The listing builds one solid part. Answer for the finished solid, in the listing's coordinates (mm). Face numbers are marked on the shaded views. A direction names the side the tool comes from. Round coordinates to 2 decimals unless told otherwise and drop trailing zeros. Loops run counter-clockwise (first coordinate to the right, second up) from the corner with the lowest first, then second, coordinate; pieces in that order, holes last. Notation, with made-up numbers: (80, 17.25) -> (125, 17.25) arc R4 cw to (125, 23.25) -> close; hole circle Ø9 at (72, 49). An arc over 180 degrees is marked (long way). Use a Markdown table: item, result. Add a question column.
Q1. For a pull along X with two mould halves and no side action, classify the marked faces 1, 2 and 3 as released by +X, released by -X, zero draft, split by the parting line, or undercut.
Q2. Which of the six approach directions +Z, -Z, +X, -X, +Y, -Y give full straight-line access (tool end or side, diameter ignored) to the marked faces 4 and 5?
Q3. Given pin 1 Ø1 at (y, z) = (185, 4.5) entering from +X; pin 2 Ø3 at (y, z) = (179.5, 3.5) entering from +X, each flat-ended and moving along its own axis, determine where each tip first touches the part or whether it passes through.
Q4. Consider line 1 (Y direction, x = 1209, z = 6); line 2 (X direction, y = 195, z = 4.5); line 3 (X direction, y = 187, z = 7). Determine where each line is inside the solid, lowest interval first.
Q5. Section A-A on x = 1208 is taken. Give the vertices of the cut face in (y, z), then the cut area to 3 significant figures.
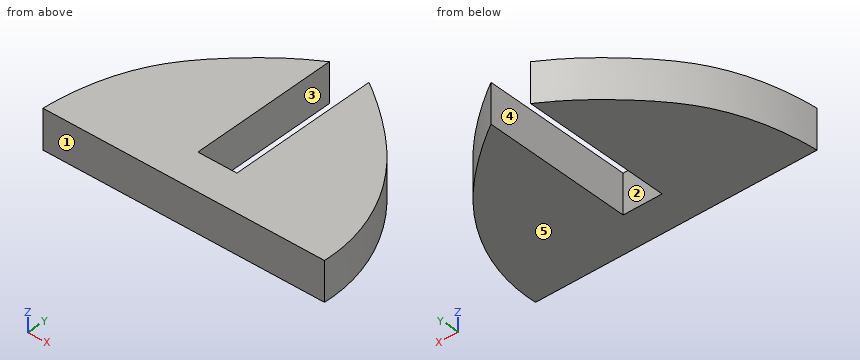
from build123d import *

# Parameters (mm, degrees)
EXTRUDE_1_DEPTH = 8


with BuildPart() as part:
    # 草图1 → 凸台-拉伸1 (new body)
    with BuildSketch(Plane.XY):
        with BuildLine():
            Line((1205.000343889, 200.380448257), (1205.000343889, 170.380448257))
            Line((1205.000343889, 170.380448257), (1212.88866118, 170.380448257))
            Line((1212.88866118, 170.380448257), (1212.88866118, 200.514821588))
            add(Edge.make_bspline(
                [(1212.88866118, 200.514821588), (1213.591796404, 200.102674546), (1216.322248426, 198.206599205), (1221.914919676, 193.964391888), (1232.595967144, 183.625439508), (1237.637966356, 171.491478384), (1237.211883134, 162.95060423)],
                knots=[0.038390069, 0.038390069, 0.038390069, 0.038390069, 0.088763706, 0.237953219, 0.477618195, 1, 1, 1, 1], degree=3))
            Line((1237.211883134, 162.95060423), (1180.232585387, 162.95060423))
            add(Edge.make_bspline(
                [(1205.000343889, 200.380448257), (1203.802132525, 199.644141671), (1199.659392578, 197.029571139), (1193.276793905, 191.438907576), (1183.524062882, 180.866285612), (1180.694379897, 169.80625417), (1180.232585387, 162.95060423)],
                knots=[0.038951436, 0.038951436, 0.038951436, 0.038951436, 0.125740292, 0.329523156, 0.570718558, 1, 1, 1, 1], degree=3))
        make_face()
    extrude(amount=EXTRUDE_1_DEPTH)


solid = part.part
Checked values:
| question | item | result |
|---|---|---|
| 1 | face 1 | zero draft |
| 1 | face 2 | undercut |
| 1 | face 3 | undercut |
| 2 | face 4 | +Z, -Z, +Y |
| 2 | face 5 | -Z, +X, -X, +Y, -Y |
| 3 | pin 1 | stops at x = 1230.38 |
| 3 | pin 2 | stops at x = 1234.13 |
| 4 | line 1 | y = 162.95 to 170.38 |
| 4 | line 2 | x = 1197.44 to 1205, 1212.89 to 1220.39 |
| 4 | line 3 | x = 1189.37 to 1205, 1212.89 to 1228.49 |
| 5 | outline | (162.95, 0) -> (170.38, 0) -> (170.38, 8) -> (162.95, 8) -> close |
| 5 | area | 59.4 mm2 |
